Read the model definition and answer for the solid it produces. Units are mm, in the model's axes. Face numbers are marked on the shaded views. A direction names the side the tool comes from. Coordinates: 2 decimals unless noted, no trailing zeros. Write each loop counter-clockwise with the first axis right and the second up, starting at its lowest first coordinate (ties: lowest second). Pieces come first, ordered by that corner, then holes. Notation, with made-up numbers: (55.5, 88) -> (67.5, 88) arc R14 ccw to (67.5, 96) -> close; hole circle Ø3 at (38.5, -20.5). An arc over 180 degrees is marked (long way). One line per item, written item: value. Start each with the question number.
1. Find section C-C, the plane z = 19.5. Write down the section's boundary in (x, y).
2. Given P1, Ø0.7, axis at y = -2, z = 6.5, coming from the +X side; P2, Ø1.7, axis at x = 0.5, z = 24.5, coming from the -Y side; P3, Ø1.2, axis at y = -1.5, z = 5.5, coming from the -X side; P4, Ø1, axis at x = -0.5, y = 0.5, coming from the -Z side, each flat-ended and moving along its own axis, determine where each tip first touches the part or whether it passes through.
3. Find section B-B, the plane z = 4.75. Write down the section's boundary in (x, y).
4. For a pull along X with two mould halves and no side action, classify the marked faces 1, 2 and 3 as pulls with the +X half, pulls with the -X half, needs draft (parallel to the pull), parting line crosses it, or undercut.
5. Consider line 1 along Z through (x, y) = (0, 0.65); line 2 along Z through (x, y) = (1.25, -2.4); line 3 along X through (y, z) = (-0.55, 8.5). Determine where each line is inside the solid, lowest interval first.
6. Find section A-A, the plane y = -2.15. Write down the section's boundary in (x, z), and give its area (3 significant figures).
7. For the marked faces 4 and 5, determine the directions among +Z, -Z, +X, -X, +Y, -Y from which every point of the face is accessible in a straight line to the end or side of a thin tool.
8. Find section D-D, the plane x = -2.5. Write down the section's boundary in (y, z).
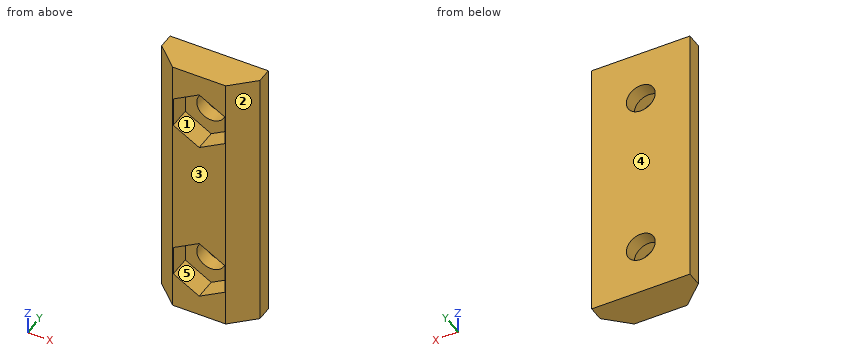
```python
from build123d import *

# Parameters (mm, degrees)
PAD_DEPTH       = 30
SKETCH001_W     = 5.88
SKETCH001_H     = 1.68
POCKET_DEPTH    = 30
POCKET001_DEPTH = 2.4
SKETCH003_R     = 1.6
POCKET002_DEPTH = 4.001


with BuildPart() as part:
    # Sketch → Pad (new body)
    with BuildSketch(Plane.XY):
        Polygon((2.94, -2.84), (-2.94, -2.84), (-5.44, -0.52), (-5.44, 1.16), (-2.94, 1.16), (-2.94, 2.84), (2.94, 2.84), (2.94, 1.16), (5.44, 1.16), (5.44, -0.52), align=None)
    extrude(amount=PAD_DEPTH)

    # Sketch001 (on Face11 of Pad) → Pocket (cut)
    with BuildSketch(Plane(origin=(0, 0, 0), x_dir=(1, 0, 0), z_dir=(0, 0, -1))):
        with Locations((0, -2)):
            Rectangle(SKETCH001_W, SKETCH001_H)
    extrude(amount=-POCKET_DEPTH, mode=Mode.SUBTRACT)

    # Sketch002 (on Face1 of Pocket) → Pocket001 (cut)
    with BuildSketch(Plane.XZ.offset(2.84)):
        Polygon((0, 27.676491), (-2.87, 26.019495), (-2.87, 22.705505), (0, 21.048509), (2.87, 22.705505), (2.87, 26.019495), align=None)
        Polygon((2.87, 7.294495), (0, 8.951491), (-2.87, 7.294495), (-2.87, 3.980505), (0, 2.323509), (2.87, 3.980505), align=None)
    extrude(amount=-POCKET001_DEPTH, mode=Mode.SUBTRACT)

    # Sketch003 (on Face21 of Pocket001) → Pocket002 (cut, through all)
    with BuildSketch(Plane(origin=(0, 1.16, 0), x_dir=(-1, 0, 0), z_dir=(0, 1, 0))):
        with Locations((0, 24.3625)):
            Circle(SKETCH003_R)
        with Locations((0, 5.6375)):
            Circle(SKETCH003_R)
    extrude(amount=-POCKET002_DEPTH, mode=Mode.SUBTRACT)


solid = part.part
```
Answer block:
1. outline: (-5.44, -0.52) -> (-2.94, -2.84) -> (2.94, -2.84) -> (5.44, -0.52) -> (5.44, 1.16) -> (-5.44, 1.16) -> close
2. P1: stops at x = 4.22
2. P2: passes through
2. P3: stops at x = -5.03
2. P4: stops at z = 0
3. outline: (-5.44, -0.52) -> (-2.94, -2.84) -> (-2.87, -2.84) -> (-2.87, -0.44) -> (-1.33, -0.44) -> (-1.33, 1.16) -> (-5.44, 1.16) -> close; (1.33, -0.44) -> (2.87, -0.44) -> (2.87, -2.84) -> (2.94, -2.84) -> (5.44, -0.52) -> (5.44, 1.16) -> (1.33, 1.16) -> close
4. face 1: undercut
4. face 2: pulls with the +X half
4. face 3: needs draft
5. line 1: z = 0 to 4.04, 7.24 to 22.76, 25.96 to 30
5. line 2: z = 0 to 3.05, 8.23 to 21.77, 26.95 to 30
5. line 3: x = -5.41 to -0.78, 0.78 to 5.41
6. outline: (-3.68, 0) -> (3.68, 0) -> (3.68, 30) -> (-3.68, 30) -> close; hole (-2.87, 3.98) -> (0, 2.32) -> (2.87, 3.98) -> (2.87, 7.29) -> (0, 8.95) -> (-2.87, 7.29) -> close; hole (-2.87, 22.71) -> (0, 21.05) -> (2.87, 22.71) -> (2.87, 26.02) -> (0, 27.68) -> (-2.87, 26.02) -> close
6. area: 164 mm2
7. face 4: +Z, -Z, +X, -X, +Y
7. face 5: -Y
8. outline: (-2.84, 0) -> (1.16, 0) -> (1.16, 30) -> (-2.84, 30) -> (-2.84, 26.23) -> (-0.44, 26.23) -> (-0.44, 22.49) -> (-2.84, 22.49) -> (-2.84, 7.51) -> (-0.44, 7.51) -> (-0.44, 3.77) -> (-2.84, 3.77) -> close
